Work out the finished part from the listing and answer in its coordinate system (mm). Face numbers are marked on the shaded views. A direction names the side the tool comes from. Coordinates: 2 decimals unless noted, no trailing zeros. Order: outer loops, then holes, each group sorted by start corner. A loop starts at its lowest first (then second) coordinate and runs counter-clockwise, first axis right, second up. Notation, with made-up numbers: (61.25, 7) - (106.25, 7) arc R18 ccw to (106.25, 37) - close; hole circle Ø1 at (85, 56). An arc over 180 degrees is marked (long way). Answer as a JSON object with one key per item and string values. Group by question number.
1) The mould has two halves that part along Z. Classify the marked faces 6, 7 and 8: released by +Z, released by -Z, zero draft, split by the parting line, or undercut.
2) Section D-D (y = 6) is taken. Give the vertices of the cut face in (x, z).
3) Each of these flat-tipped pins is pushed along its axis until it touches: P1, Ø4, axis at x = -6, z = 14.5, coming from the +Y side; P2, Ø8, axis at x = 9, z = 8.5, coming from the +Y side; P3, Ø6, axis at x = -7.5, z = 6.5, coming from the -Y side; P4, Ø2.5, axis at x = 0, y = 0, coming from the -Z side. Where does it stop, or does it pass through?
4) A tool of negligible diameter and unlimited length cuts with its end or side. For the marked faces 1, 2, 3, 4 and 5, from which of +Z, -Z, +X, -X, +Y, -Y can it reach the whole face along a straight path? Write none if from no direction.
5) Section A-A (y = 0) is taken. Give the vertices of the cut face in (x, z), plus the area to 3 significant figures.
6) Find the intervals of material crossed by line 1 along X through (y, z) = (8.25, 0.5); line 2 along Y through (x, z) = (0, 11.7); line 3 along Z through (x, y) = (-1.75, 11.75), in increasing order.
7) Section C-C (x = 5.25) is taken. Give the vertices of the cut face in (y, z), plus the area to 3 significant figures.
Autodesk Inventor part; units mm, degrees
ref_plane "YZ Plane" through (0, 0, 0) normal (1, 0, 0) x (0, 1, 0)
ref_plane "XZ Plane" through (0, 0, 0) normal (0, 1, 0) x (-1, 0, 0)
ref_plane "XY Plane" through (0, 0, 0) normal (0, 0, 1) x (1, 0, 0)
sketch "Skizze1" plane through (0, 0, 0) normal (0, 0, 1) x (1, 0, 0)
  circle A0 centre (0, 0) radius 9.99
  dimension "d0" = 19.98
extrude "Extrusion1" add sketch "Skizze1" along normal blind 15
sketch "Skizze2" plane through (0, 0, 15) normal (0, 0, 1) x (1, 0, 0)
  circle A0 centre (0, 0) radius 9.99
  line L0 (-0.5, 9.9775) -> (0.5, 9.9775)
  line L1 (-0.5, 9.9775) -> (-0.5177, 11.3774)
  line L2 (0.4823, 11.3774) -> (0.5, 9.9775)
  line L3 (-0.5177, 11.3774) -> (-0.419, 11.4786)
  line L4 (0.381, 11.4786) -> (0.4823, 11.3774)
  line L5 (-0.419, 11.4786) -> (0.381, 11.4786)
  line L6 (-4.2802, 9.0266) -> (-4.8322, 10.3132)
  line L7 (-4.8322, 10.3132) -> (-4.7798, 10.4445)
  line L8 (-4.7798, 10.4445) -> (-4.0407, 10.7507)
  line L9 (-4.0407, 10.7507) -> (-3.9084, 10.6959)
  line L10 (-3.9084, 10.6959) -> (-3.3563, 9.4093)
  line L11 (-4.2802, 9.0266) -> (-3.3563, 9.4093)
  line L12 (-7.4087, 6.7016) -> (-8.4111, 7.6789)
  line L13 (-8.4111, 7.6789) -> (-8.4129, 7.8203)
  line L14 (-8.4129, 7.8203) -> (-7.8472, 8.386)
  line L15 (-7.8472, 8.386) -> (-7.704, 8.386)
  line L16 (-7.704, 8.386) -> (-6.7016, 7.4087)
  line L17 (-7.4087, 6.7016) -> (-6.7016, 7.4087)
  line L18 (-9.4093, 3.3563) -> (-10.7094, 3.8756)
  line L19 (-10.7094, 3.8756) -> (-10.7652, 4.0056)
  line L20 (-10.7652, 4.0056) -> (-10.4591, 4.7447)
  line L21 (-10.4591, 4.7447) -> (-10.3268, 4.7995)
  line L22 (-10.3268, 4.7995) -> (-9.0266, 4.2802)
  line L23 (-9.4093, 3.3563) -> (-9.0266, 4.2802)
  line L24 (-9.9775, -0.5) -> (-11.3774, -0.5177)
  line L25 (-11.3774, -0.5177) -> (-11.4786, -0.419)
  line L26 (-11.4786, -0.419) -> (-11.4786, 0.381)
  line L27 (-11.4786, 0.381) -> (-11.3774, 0.4823)
  line L28 (-11.3774, 0.4823) -> (-9.9775, 0.5)
  line L29 (-9.9775, -0.5) -> (-9.9775, 0.5)
  line L30 (-9.0266, -4.2802) -> (-10.3132, -4.8322)
  line L31 (-10.3132, -4.8322) -> (-10.4445, -4.7798)
  line L32 (-10.4445, -4.7798) -> (-10.7507, -4.0407)
  line L33 (-10.7507, -4.0407) -> (-10.6959, -3.9084)
  line L34 (-10.6959, -3.9084) -> (-9.4093, -3.3563)
  line L35 (-9.0266, -4.2802) -> (-9.4093, -3.3563)
  line L36 (-6.7016, -7.4087) -> (-7.6789, -8.4111)
  line L37 (-7.6789, -8.4111) -> (-7.8203, -8.4129)
  line L38 (-7.8203, -8.4129) -> (-8.386, -7.8472)
  line L39 (-8.386, -7.8472) -> (-8.386, -7.704)
  line L40 (-8.386, -7.704) -> (-7.4087, -6.7016)
  line L41 (-6.7016, -7.4087) -> (-7.4087, -6.7016)
  line L42 (-3.3563, -9.4093) -> (-3.8756, -10.7094)
  line L43 (-3.8756, -10.7094) -> (-4.0056, -10.7652)
  line L44 (-4.0056, -10.7652) -> (-4.7447, -10.4591)
  line L45 (-4.7447, -10.4591) -> (-4.7995, -10.3268)
  line L46 (-4.7995, -10.3268) -> (-4.2802, -9.0266)
  line L47 (-3.3563, -9.4093) -> (-4.2802, -9.0266)
  line L48 (0.5, -9.9775) -> (0.5177, -11.3774)
  line L49 (0.5177, -11.3774) -> (0.419, -11.4786)
  line L50 (0.419, -11.4786) -> (-0.381, -11.4786)
  line L51 (-0.381, -11.4786) -> (-0.4823, -11.3774)
  line L52 (-0.4823, -11.3774) -> (-0.5, -9.9775)
  line L53 (0.5, -9.9775) -> (-0.5, -9.9775)
  line L54 (4.2802, -9.0266) -> (4.8322, -10.3132)
  line L55 (4.8322, -10.3132) -> (4.7798, -10.4445)
  line L56 (4.7798, -10.4445) -> (4.0407, -10.7507)
  line L57 (4.0407, -10.7507) -> (3.9084, -10.6959)
  line L58 (3.9084, -10.6959) -> (3.3563, -9.4093)
  line L59 (4.2802, -9.0266) -> (3.3563, -9.4093)
  line L60 (7.4087, -6.7016) -> (8.4111, -7.6789)
  line L61 (8.4111, -7.6789) -> (8.4129, -7.8203)
  line L62 (8.4129, -7.8203) -> (7.8472, -8.386)
  line L63 (7.8472, -8.386) -> (7.704, -8.386)
  line L64 (7.704, -8.386) -> (6.7016, -7.4087)
  line L65 (7.4087, -6.7016) -> (6.7016, -7.4087)
  line L66 (9.4093, -3.3563) -> (10.7094, -3.8756)
  line L67 (10.7094, -3.8756) -> (10.7652, -4.0056)
  line L68 (10.7652, -4.0056) -> (10.4591, -4.7447)
  line L69 (10.4591, -4.7447) -> (10.3268, -4.7995)
  line L70 (10.3268, -4.7995) -> (9.0266, -4.2802)
  line L71 (9.4093, -3.3563) -> (9.0266, -4.2802)
  line L72 (9.9775, 0.5) -> (11.3774, 0.5177)
  line L73 (11.3774, 0.5177) -> (11.4786, 0.419)
  line L74 (11.4786, 0.419) -> (11.4786, -0.381)
  line L75 (11.4786, -0.381) -> (11.3774, -0.4823)
  line L76 (11.3774, -0.4823) -> (9.9775, -0.5)
  line L77 (9.9775, 0.5) -> (9.9775, -0.5)
  line L78 (9.0266, 4.2802) -> (10.3132, 4.8322)
  line L79 (10.3132, 4.8322) -> (10.4445, 4.7798)
  line L80 (10.4445, 4.7798) -> (10.7507, 4.0407)
  line L81 (10.7507, 4.0407) -> (10.6959, 3.9084)
  line L82 (10.6959, 3.9084) -> (9.4093, 3.3563)
  line L83 (9.0266, 4.2802) -> (9.4093, 3.3563)
  line L84 (6.7016, 7.4087) -> (7.6789, 8.4111)
  line L85 (7.6789, 8.4111) -> (7.8203, 8.4129)
  line L86 (7.8203, 8.4129) -> (8.386, 7.8472)
  line L87 (8.386, 7.8472) -> (8.386, 7.704)
  line L88 (8.386, 7.704) -> (7.4087, 6.7016)
  line L89 (6.7016, 7.4087) -> (7.4087, 6.7016)
  line L90 (3.3563, 9.4093) -> (3.8756, 10.7094)
  line L91 (3.8756, 10.7094) -> (4.0056, 10.7652)
  line L92 (4.0056, 10.7652) -> (4.7447, 10.4591)
  line L93 (4.7447, 10.4591) -> (4.7995, 10.3268)
  line L94 (4.7995, 10.3268) -> (4.2802, 9.0266)
  line L95 (3.3563, 9.4093) -> (4.2802, 9.0266)
  dimension "d4" = 1
  dimension "d31" = 0.1
  dimension "d52" = 360
extrude "Extrusion2" add sketch "Skizze2" against normal blind 15 contours A0 L72 L73 L74 L75 L76 | A0 L78 L79 L80 L81 L82 | L66 L67 L68 L69 L70 A0 | A0 L71 | A0 L84 L85 L86 L87 L88 | L60 L61 L62 L63 L64 A0 | A0 L65 | A0 L90 L91 L92 L93 L94 | L54 L55 L56 L57 L58 A0 | A0 L59 | L0 A0 | A0 L1 L3 L5 L4 L2 | L48 L49 L50 L51 L52 A0 | A0 L53 | A0 L6 L7 L8 L9 L10 | L42 L43 L44 L45 L46 A0 | A0 L12 L13 L14 L15 L16 | L36 L37 L38 L39 L40 A0 | L23 A0 | A0 L18 L19 L20 L21 L22 | L30 L31 L32 L33 L34 A0 | A0 L35 | L29 A0 | A0 L24 L25 L26 L27 L28
sketch "Skizze3" plane through (0, 0, 15) normal (0, 0, 1) x (1, 0, 0)
  circle A0 centre (0, 0) radius 12.5
  dimension "d15" = 25
extrude "Extrusion3" add sketch "Skizze3" along normal blind 1.5
sketch "Skizze4" plane through (0, 0, 0) normal (0, 0, -1) x (-1, 0, 0)
  circle A0 centre (0, 0) radius 12.5
  dimension "d33" = 25
extrude "Extrusion4" add sketch "Skizze4" along normal blind 1.5
sketch "Skizze5" plane through (0, 0, 16.5) normal (0, 0, 1) x (1, 0, 0)
  circle A0 centre (0, 0) radius 2.75
  dimension "d20" = 5.5
extrude "Extrusion5" cut sketch "Skizze5" against normal blind 3.5
sketch "Skizze6" plane through (0, 0, -1.5) normal (0, 0, -1) x (-1, 0, 0)
  circle A0 centre (0, 0) radius 2.75
  dimension "d23" = 5.5
extrude "Extrusion6" cut sketch "Skizze6" against normal blind 12
sketch "Skizze7" plane through (0, 0, 10.5) normal (0, 0, -1) x (-1, 0, 0)
  circle A0 centre (0, 0) radius 1.6
  dimension "d26" = 3.2
extrude "Extrusion7" cut sketch "Skizze7" against normal blind 12
properties part number "zahnrad2"
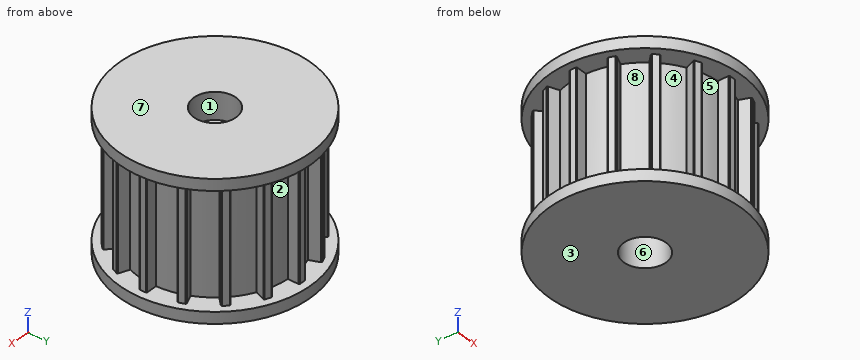
Report:
{
 "1": {"face 6": "zero draft", "face 7": "released by +Z", "face 8": "undercut"},
 "2": {"outline": "(-10.97, -1.5) - (10.97, -1.5) - (10.97, 0) - (7.99, 0) - (7.99, 15) - (10.97, 15) - (10.97, 16.5) - (-10.97, 16.5) - (-10.97, 15) - (-7.99, 15) - (-7.99, 0) - (-10.97, 0) - close"},
 "3": {"P1": "stops at y = 11.82", "P2": "stops at y = 8.65", "P3": "stops at y = -10.56", "P4": "passes through"},
 "4": {"face 1": "+Z", "face 2": "+Y", "face 3": "-Z, +X, -X, +Y, -Y", "face 4": "none", "face 5": "-Y"},
 "5": {"outline": "(-12.5, -1.5) - (-2.75, -1.5) - (-2.75, 10.5) - (-1.6, 10.5) - (-1.6, 13) - (-2.75, 13) - (-2.75, 16.5) - (-12.5, 16.5) - (-12.5, 15) - (-11.48, 15) - (-11.48, 0) - (-12.5, 0) - close; (1.6, 10.5) - (2.75, 10.5) - (2.75, -1.5) - (12.5, -1.5) - (12.5, 0) - (11.48, 0) - (11.48, 15) - (12.5, 15) - (12.5, 16.5) - (2.75, 16.5) - (2.75, 13) - (1.6, 13) - close", "area": "326 mm²"},
 "6": {"line 1": "x = -7.98 to -7.56, -5.63 to 5.63, 7.52 to 7.98", "line 2": "y = -11.48 to -1.6, 1.6 to 11.48", "line 3": "z = -1.5 to 0, 15 to 16.5"},
 "7": {"outline": "(-11.34, -1.5) - (11.34, -1.5) - (11.34, 0) - (8.5, 0) - (8.5, 15) - (11.34, 15) - (11.34, 16.5) - (-11.34, 16.5) - (-11.34, 15) - (-8.5, 15) - (-8.5, 0) - (-11.34, 0) - close", "area": "323 mm²"}
}
